Verification items for the finished model (mm, model axes). Face numbers are marked on the shaded views. A direction names the side the tool comes from. Coordinates: 2 decimals unless noted, no trailing zeros. Order: outer loops, then holes, each group sorted by start corner. A loop starts at its lowest first (then second) coordinate and runs counter-clockwise, first axis right, second up. Notation, with made-up numbers: (56.25, 74) - (112.25, 74) arc R19 ccw to (112.25, 110) - close; hole circle Ø4 at (4.5, 11.5). An arc over 180 degrees is marked (long way). Answer as CSV lines item,"result". Start each with the question number.
1. Go/stop test with flat-tipped pins: pin 1 (0.9 mm diameter, centred on x = 6, z = 17, fed in from -Y); pin 2 (0.7 mm diameter, centred on y = -1.5, z = 9.5, fed in from -X); pin 3 (4 mm diameter, centred on x = -1, z = 17, fed in from +Y). Record where each tip stops, or that it passes through.
2. Set-up check for the marked faces 1 and 2: record each of +Z, -Z, +X, -X, +Y, -Y from which the full face is reachable in a straight line by a thin tool's end or side.
3. Section check B-B (x = -1.75). Record the cut outline in (y, z), and give its area (3 significant figures).
4. Material ranges on L1, parallel to X at y = 1.05, z = 22; L2, parallel to Y at x = -5, z = 22; L3, parallel to Y at x = -1, z = 16, recorded low to high. Write a range as [from, to].
5. Section check D-D (x = -5.75). Record the cut outline in (y, z).
6. Section check A-A (y = 1.65). Record the cut outline in (x, z).
from build123d import *

# Parameters (mm, degrees)
AUFSATZ_LINEAR_AUSTRAGEN1_DEPTH = 25
SKIZZE2_W                       = 6
SKIZZE2_H                       = 1.8
AUFSATZ_LINEAR_AUSTRAGEN2_DEPTH = 8
SKIZZE3_W                       = 7.5
SKIZZE3_H                       = 0.65
SCHNITT_LINEAR_AUSTRAGEN1_DEPTH = 34
VERRUNDUNG1_R                   = 0.2


with BuildPart() as part:
    # Skizze1 → Aufsatz-Linear austragen1 (new body)
    with BuildSketch(Plane.XY):
        Polygon((-4.75, 0.9), (-6.7, 0.9), (-6.7, -0.9), (-4.75, -0.9), (-4.75, -2.9), (-3.75, -2.9), (-3.75, -0.9), (3.75, -0.9), (3.75, -2.9), (4.75, -2.9), (4.75, -0.9), (6.7, -0.9), (6.7, 0.9), (4.75, 0.9), (4.75, 2.9), (3.75, 2.9), (3.75, 0.9), (-3.75, 0.9), (-3.75, 2.9), (-4.75, 2.9), align=None)
    extrude(amount=AUFSATZ_LINEAR_AUSTRAGEN1_DEPTH)

    # Skizze2 → Aufsatz-Linear austragen2 (add)
    with BuildSketch(Plane(origin=(0, 0, 0), x_dir=(-1, 0, 0), z_dir=(0, 0, -1))):
        Rectangle(SKIZZE2_W, SKIZZE2_H)
    extrude(amount=AUFSATZ_LINEAR_AUSTRAGEN2_DEPTH)

    # Skizze3 → Schnitt-Linear austragen1 (cut, through all)
    with BuildSketch(Plane.XY.offset(25)):
        with Locations((0, -0.575)):
            Rectangle(SKIZZE3_W, SKIZZE3_H)
        with Locations((0, 0.575)):
            Rectangle(SKIZZE3_W, SKIZZE3_H)
    extrude(amount=-SCHNITT_LINEAR_AUSTRAGEN1_DEPTH, mode=Mode.SUBTRACT)

    # Verrundung1
    verrundung1_edges = [part.edges().sort_by_distance(p)[0] for p in [
        (0, 0.25, 25),
        (-4.75, -1.9, 25),
        (-4.25, -2.9, 25),
        (-5.725, 0.9, 0),
        (-4.75, 1.9, 0),
        (-4.25, 2.9, 0),
        (-3.75, -1.575, 25),
        (4.25, 2.9, 0),
        (4.75, 1.9, 0),
        (5.725, 0.9, 0),
        (6.7, 0, 0),
        (5.725, -0.9, 0),
        (4.75, -1.9, 0),
        (4.25, -2.9, 0),
        (-4.25, -2.9, 0),
        (-4.75, -1.9, 0),
        (-5.725, -0.9, 0),
        (-6.7, 0, 0),
        (3.75, -1.575, 25),
        (4.25, -2.9, 25),
        (-6.7, 0.9, 12.5),
        (-4.75, 2.9, 12.5),
        (-3.75, 2.9, 12.5),
        (3.75, 2.9, 12.5),
        (4.75, 2.9, 12.5),
        (6.7, 0.9, 12.5),
        (6.7, -0.9, 12.5),
        (4.75, -2.9, 12.5),
        (3.75, -2.9, 12.5),
        (-3.75, -2.9, 12.5),
        (-4.75, -2.9, 12.5),
        (-6.7, -0.9, 12.5),
        (4.75, -1.9, 25),
        (5.725, -0.9, 25),
        (6.7, 0, 25),
        (5.725, 0.9, 25),
        (-6.7, 0, 25),
        (4.75, 1.9, 25),
        (4.25, 2.9, 25),
        (3.75, 1.575, 25),
        (-3.75, 1.575, 25),
        (3, 0, -8),
        (-3, 0, -8),
        (-4.25, 2.9, 25),
        (0, 0.25, -8),
        (0, -0.25, -8),
        (-4.75, 1.9, 25),
        (-5.725, 0.9, 25),
        (0, -0.25, 25),
        (-5.725, -0.9, 25),
    ]]
    fillet(verrundung1_edges, radius=VERRUNDUNG1_R)


solid = part.part
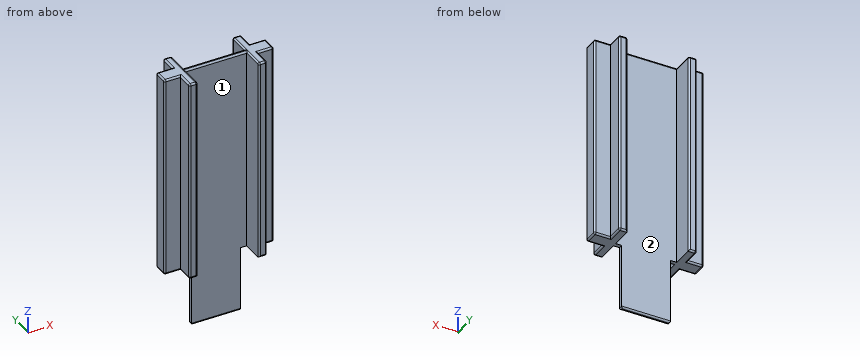
Evaluation:
1,pin 1,"stops at y = -0.9"
1,pin 2,"stops at x = -4.75"
1,pin 3,"stops at y = 0.25"
2,face 1,"+Z, -Z, -Y"
2,face 2,"+Z, -Z, +Y"
3,outline,"(-0.25, -7.8) arc R0.2 ccw to (-0.05, -8) - (0.05, -8) arc R0.2 ccw to (0.25, -7.8) - (0.25, 24.8) arc R0.2 ccw to (0.05, 25) - (-0.05, 25) arc R0.2 ccw to (-0.25, 24.8) - close"
3,area,"16.5 mm²"
4,L1,"x = [-4.75, -3.75], [3.75, 4.75]"
4,L2,"y = [-0.9, 0.9]"
4,L3,"y = [-0.25, 0.25]"
5,outline,"(-0.9, 0.2) arc R0.2 ccw to (-0.7, 0) - (0.7, 0) arc R0.2 ccw to (0.9, 0.2) - (0.9, 24.8) arc R0.2 ccw to (0.7, 25) - (-0.7, 25) arc R0.2 ccw to (-0.9, 24.8) - close"
6,outline,"(-4.75, 0.2) arc R0.2 ccw to (-4.55, 0) - (-3.75, 0) - (-3.75, 24.8) arc R0.2 ccw to (-3.95, 25) - (-4.55, 25) arc R0.2 ccw to (-4.75, 24.8) - close; (3.75, 0) - (4.55, 0) arc R0.2 ccw to (4.75, 0.2) - (4.75, 24.8) arc R0.2 ccw to (4.55, 25) - (3.95, 25) arc R0.2 ccw to (3.75, 24.8) - close"
